Source: CAD feature listing. Evaluate the final solid. Frame: model axes, mm. A direction names the side the tool comes from. Round coordinates to 2 decimals unless told otherwise and drop trailing zeros. Order: outer loops, then holes, each group sorted by start corner. A loop starts at its lowest first (then second) coordinate and runs counter-clockwise, first axis right, second up. Notation, with made-up numbers: (35.5, -16) -> (74.5, -16) arc R20 ccw to (74.5, -12) -> close; hole circle Ø10 at (74, 73). An arc over 180 degrees is marked (long way). One line per item, written item: value. Start each with the question number.
1) Mould query, pull axis Y, two halves, no side actions, for faces 3 (the face through (8, 6, 9)), 4 (the face through (10, 5, 11)), 5 (the face through (0, 16, 11)), 6 (the face through (-3, 0, 2)). Classes: pulls with the +Y half, pulls with the -Y half, needs draft (parallel to the pull), parting line crosses it, or undercut.
2) Section D-D (z = 16.5). Return the cut outline in (x, y).
3) Section A-A (y = 1.5). Return the cut outline in (x, z).
4) Pin query (flat end, axial travel): P1, Ø1, axis at x = 0.5, y = 0, coming from the +Z side; P2, Ø6, axis at x = 3, z = 15.5, coming from the -Y side; P3, Ø4, axis at x = -7, z = 16, coming from the -Y side; P4, Ø4, axis at x = 0, y = 3, coming from the +Z side. Return the tip coordinate at first contact, or that it passes through.
5) Section C-C (x = 1.25). Return the cut outline in (y, z).
6) Section B-B (z = 9.25). Return the cut outline in (x, y).
7) Reachability of faces 1 (the face through (2, 12, 13)), 2 (the face through (-10, 5, 11)) from +Z, -Z, +X, -X, +Y, -Y: full face, straight path, thin tool, end or side. Return the list, or none.
8) Ray query, L1, parallel to X at y = 14.15, z = 16; L2, parallel to Y at x = 0, z = 2.45; L3, parallel to Z at x = 0, y = 13.8. Return the intervals inside material, ascending.
```python
from build123d import *

# Parameters (mm, degrees)
F0_W     = 24
F0_H     = 24
F0_R     = 3
F1_DEPTH = 4
F3_DEPTH = 28
F5_DEPTH = 25
F6_SIZE  = 10
F7_W     = 4
F7_H     = 14
F8_DEPTH = 14
F9_SIZE  = 13.99999


# Not quite as in the source:
# - a fillet or chamfer is up to 0.001 mm smaller than in the source, because OpenCascade refuses the exact size


with BuildPart() as f1:
    # F0 (on Top) → F1 (new body)
    with BuildSketch(Plane.XY):
        Rectangle(F0_W, F0_H)
        Circle(F0_R, mode=Mode.SUBTRACT)
    extrude(amount=F1_DEPTH)

    # F2 (on Top) → F3 (join)
    with BuildSketch(Plane.XY):
        Polygon((-12.0000001043, 12), (0, 12), (11.9999998957, 12), (11.9999998957, 16), (-12.0000001043, 16), align=None)
    extrude(amount=F3_DEPTH)

    # F4 (on face) → F5 (cut)
    with BuildSketch(Plane.XZ.offset(-12)):
        with BuildLine():
            ThreePointArc((0, 13), (2.1213203436, 13.8786796564), (3, 16))
            ThreePointArc((3, 16), (-2.1213203436, 18.1213203436), (0, 13))
        make_face()
    extrude(amount=-F5_DEPTH, mode=Mode.SUBTRACT)

    # F6
    f6_edges = [f1.edges().sort_by_distance(p)[0] for p in [
        (-12, -12, 2),
        (12, -12, 2),
        (-12, 14, 28),
        (12, 14, 28),
    ]]
    chamfer(f6_edges, length=F6_SIZE)

    # F7 (on face) → F8 (join)
    with BuildSketch(Plane.XY.offset(4)):
        with Locations((-10, 5)):
            Rectangle(F7_W, F7_H)
        with Locations((10, 5)):
            Rectangle(F7_W, F7_H)
    extrude(amount=F8_DEPTH)

    # F9 (size 14 in the source; OpenCascade refuses exactly that, so slightly less here)
    f9_edges = [f1.edges().sort_by_distance(p)[0] for p in [
        (-10, -2, 18),
        (10, -2, 18),
    ]]
    chamfer(f9_edges, length=F9_SIZE)


solid = f1.part
```
Findings:
1. face 3: needs draft
1. face 4: pulls with the -Y half
1. face 5: pulls with the +Y half
1. face 6: undercut
2. outline: (-12, 10.5) -> (-8, 10.5) -> (-8, 12) -> (-2.96, 12) -> (-2.96, 16) -> (-12, 16) -> close; (2.96, 12) -> (8, 12) -> (8, 10.5) -> (12, 10.5) -> (12, 16) -> (2.96, 16) -> close
3. outline: (-12, 0) -> (-2.6, 0) -> (-2.6, 4) -> (-8, 4) -> (-8, 7.5) -> (-12, 7.5) -> close; (2.6, 0) -> (12, 0) -> (12, 7.5) -> (8, 7.5) -> (8, 4) -> (2.6, 4) -> close
4. P1: through
4. P2: y = 12
4. P3: y = 8.27
4. P4: z = 4
5. outline: (-12, 0) -> (-2.73, 0) -> (-2.73, 4) -> (-12, 4) -> close; (2.73, 0) -> (16, 0) -> (16, 13.27) -> (12, 13.27) -> (12, 4) -> (2.73, 4) -> close; (12, 18.73) -> (16, 18.73) -> (16, 28) -> (12, 28) -> close
6. outline: (-12, 3.25) -> (-8, 3.25) -> (-8, 12) -> (8, 12) -> (8, 3.25) -> (12, 3.25) -> (12, 16) -> (-12, 16) -> close
7. face 1: +Z, -Y
7. face 2: +Z, +X, -X, -Y
8. L1: -12 to -3, 3 to 12
8. L2: -12 to -3, 3 to 16
8. L3: 0 to 13, 19 to 28
